Autodesk Inventor part; units mm, degrees
ref_plane "YZ Plane" through (0, 0, 0) normal (1, 0, 0) x (0, 1, 0)
ref_plane "XZ Plane" through (0, 0, 0) normal (0, 1, 0) x (-1, 0, 0)
ref_plane "XY Plane" through (0, 0, 0) normal (0, 0, 1) x (1, 0, 0)
sketch "스케치1" plane through (0, 0, 0) normal (0, 1, 0) x (-1, 0, 0)
  line L0 (-62.3615, 62.3615) -> (-22.8259, 85.1874)
  line L1 (-22.8259, 85.1874) -> (22.8259, 85.1874)
  line L2 (22.8259, 85.1874) -> (62.3615, 62.3615)
  line L3 (62.3615, 62.3615) -> (85.1874, 22.8259)
  line L4 (85.1874, 22.8259) -> (85.1874, -22.8259)
  line L5 (85.1874, -22.8259) -> (62.3615, -62.3615)
  line L6 (62.3615, -62.3615) -> (22.8259, -85.1874)
  line L7 (22.8259, -85.1874) -> (-22.8259, -85.1874)
  line L8 (-22.8259, -85.1874) -> (-62.3615, -62.3615)
  line L9 (-62.3615, -62.3615) -> (-85.1874, -22.8259)
  line L10 (-85.1874, -22.8259) -> (-85.1874, 22.8259)
  line L11 (-85.1874, 22.8259) -> (-62.3615, 62.3615)
  line L12 (88.3874, -23.6833) -> (64.7041, -64.7041)
  line L13 (64.7041, -64.7041) -> (23.6833, -88.3874)
  line L14 (23.6833, -88.3874) -> (-23.6833, -88.3874)
  line L15 (-23.6833, -88.3874) -> (-64.7041, -64.7041)
  line L16 (-64.7041, -64.7041) -> (-88.3874, -23.6833)
  line L17 (-88.3874, -23.6833) -> (-88.3874, 23.6833)
  line L18 (-88.3874, 23.6833) -> (-64.7041, 64.7041)
  line L19 (-64.7041, 64.7041) -> (-23.6833, 88.3874)
  line L20 (-23.6833, 88.3874) -> (23.6833, 88.3874)
  line L21 (23.6833, 88.3874) -> (64.7041, 64.7041)
  line L22 (64.7041, 64.7041) -> (88.3874, 23.6833)
  line L23 (88.3874, 23.6833) -> (88.3874, -23.6833)
  point P0 (0, 0)
  point P1 (0, 0)
  point P2 (0, 0)
  dimension "d0" = 176.385
  dimension "d1" = 3.2
extrude "돌출1" add sketch "스케치1" along normal blind 6.8 contours L0 L1 L2 L3 L4 L5 L6 L7 L8 L9 L10 L11 | L12 L13 L14 L15 L16 L17 L18 L19 L20 L21 L22 L23
sketch "스케치2" plane through (0, 6.8, 0) normal (0, 1, 0) x (1, 0, 0)
  line L0 (-23.2546, 86.7874) -> (23.2546, 86.7874)
  line L1 (23.2546, 86.7874) -> (63.5328, 63.5328)
  line L2 (63.5328, 63.5328) -> (86.7874, 23.2546)
  line L3 (86.7874, 23.2546) -> (86.7874, -23.2546)
  line L4 (86.7874, -23.2546) -> (63.5328, -63.5328)
  line L5 (63.5328, -63.5328) -> (23.2546, -86.7874)
  line L6 (23.2546, -86.7874) -> (-23.2546, -86.7874)
  line L7 (-23.2546, -86.7874) -> (-63.5328, -63.5328)
  line L8 (-63.5328, -63.5328) -> (-86.7874, -23.2546)
  line L9 (-86.7874, -23.2546) -> (-86.7874, 23.2546)
  line L10 (-86.7874, 23.2546) -> (-63.5328, 63.5328)
  line L11 (-63.5328, 63.5328) -> (-23.2546, 86.7874)
  line L12 (-88.3874, 23.6833) -> (-88.3874, -23.6833)
  line L13 (22.7187, -84.7874) -> (-22.7187, -84.7874)
  line L14 (-22.7187, -84.7874) -> (-62.0687, -62.0687)
  line L15 (-62.0687, -62.0687) -> (-84.7874, -22.7187)
  line L16 (-84.7874, -22.7187) -> (-84.7874, 22.7187)
  line L17 (-84.7874, 22.7187) -> (-62.0687, 62.0687)
  line L18 (-62.0687, 62.0687) -> (-22.7187, 84.7874)
  line L19 (-22.7187, 84.7874) -> (22.7187, 84.7874)
  line L20 (22.7187, 84.7874) -> (62.0687, 62.0687)
  line L21 (62.0687, 62.0687) -> (84.7874, 22.7187)
  line L22 (84.7874, 22.7187) -> (84.7874, -22.7187)
  line L23 (84.7874, -22.7187) -> (62.0687, -62.0687)
  line L24 (62.0687, -62.0687) -> (22.7187, -84.7874)
  point P0 (0, 0)
  point P1 (0, 0)
  point P2 (0, 0)
  dimension "d4" = 1.6
  dimension "d5" = 2
extrude "돌출2" cut sketch "스케치2" against normal blind 1.2
sketch "스케치5" plane through (0, 6.8, 0) normal (0, 1, 0) x (1, 0, 0)
  line L0 (-62.0687, -62.0687) -> (-22.7187, -84.7874)
  line L1 (-22.7187, -84.7874) -> (22.7187, -84.7874)
  line L2 (22.7187, -84.7874) -> (62.0687, -62.0687)
  line L3 (62.0687, -62.0687) -> (84.7874, -22.7187)
  line L4 (84.7874, -22.7187) -> (84.7874, 22.7187)
  line L5 (84.7874, 22.7187) -> (62.0687, 62.0687)
  line L6 (62.0687, 62.0687) -> (22.7187, 84.7874)
  line L7 (22.7187, 84.7874) -> (-22.7187, 84.7874)
  line L8 (-22.7187, 84.7874) -> (-62.0687, 62.0687)
  line L9 (-62.0687, 62.0687) -> (-84.7874, 22.7187)
  line L10 (-84.7874, 22.7187) -> (-84.7874, -22.7187)
  line L11 (-84.7874, -22.7187) -> (-62.0687, -62.0687)
  point P0 (0, 0)
extrude "돌출5" cut sketch "스케치5" against normal blind 0.6
fillet "모깎기1" radius 1.2 24 edges at (76.5457, 0, 44.1937) (76.5457, 6.8, 44.1937) (88.3874, 6.8, 0) (88.3874, 0, 0) (76.5457, 6.8, -44.1937) (76.5457, 0, -44.1937) (44.1937, 6.8, -76.5457) (44.1937, 0, -76.5457) (0, 0, -88.3874) (0, 6.8, -88.3874) (-44.1937, 6.8, -76.5457) (-44.1937, 0, -76.5457) (-76.5457, 0, -44.1937) (-76.5457, 6.8, -44.1937) (-88.3874, 0, 0) (-88.3874, 6.8, 0) (-76.5457, 0, 44.1937) (-76.5457, 6.8, 44.1937) (-44.1937, 0, 76.5457) (-44.1937, 6.8, 76.5457) (0, 0, 88.3874) (0, 6.8, 88.3874) (44.1937, 0, 76.5457) (44.1937, 6.8, 76.5457)
sketch "스케치7" plane through (0, 0, 0) normal (0, -1, 0) x (1, 0, 0)
  line L0 (10, -7.5) -> (-10, -7.5)
  line L1 (-10, -7.5) -> (-10, -2.5)
  line L2 (-10, -2.5) -> (10, -2.5)
  line L3 (10, -2.5) -> (10, -7.5)
  line L4 (10, -7.5) -> (-10, -2.5) construction
  line L5 (-10, -7.5) -> (10, -2.5) construction
  line L6 (0, 0) -> (-24.3026, 0)
  line L7 (10, 7.5) -> (-10, 7.5)
  line L8 (-10, 7.5) -> (-10, 2.5)
  line L9 (-10, 2.5) -> (10, 2.5)
  line L10 (10, 2.5) -> (10, 7.5)
  line L11 (10, 7.5) -> (-10, 2.5) construction
  line L12 (-10, 7.5) -> (10, 2.5) construction
  point P0 (0, -5)
  point P1 (0, 5)
  dimension "d26" = 20
  dimension "d27" = 5
  dimension "d28" = 2.5
extrude "돌출7" add sketch "스케치7" along normal blind 10
sketch "스케치8" plane through (-10, 0, 7.5) normal (0, 0, 1) x (1, 0, 0)
  circle A0 centre (15, -5) radius 1.25
  line L0 (-13.3618, 0) -> (33.3618, 0)
  line L1 (20, 0) -> (20, -10)
  line L2 (20, -10) -> (0, -10)
  line L3 (10, -10) -> (10, 0)
  circle A1 centre (5, -5) radius 1.25
  point P0 (20, -5)
  dimension "d31" = 2.5
  dimension "d32" = 5
  dimension "d33" = 5
extrude "돌출8" cut sketch "스케치8" against normal up to surface (15 mm away) contours A0 | A1
properties part number "(x2)_POSPA_Large_Bottom"
Build history of the part. All positions in model axes, mm. A direction names the side the tool comes from. Give positions to 0.01 mm unless a question says otherwise; leave off trailing zeros. Use a Markdown table: item, result.
(1) Wall check: line 1 along Y through (x, z) = (-5, 3); line 2 along Z through (x, y) = (28.5, 5.75); line 3 along Z through (x, y) = (8.5, -0.75). Give the ranges that are in metal, low to high.
Taken from the geometry:
| item | result |
|---|---|
| line 1 | -10 to -6.25, -3.75 to 6.2 |
| line 2 | -85.6 to -83.76, -81.45 to 81.45, 83.76 to 85.6 |
| line 3 | -7.5 to -2.5, 2.5 to 7.5 |
(2) Drop flat-ended pins along their axis: pin 1 Ø1.5 at (y, z) = (-3.5, 6) entering from +X; pin 2 Ø1 at (x, y) = (7.5, 6.5) entering from -Z; pin 3 Ø5 at (x, y) = (-1.5, -4) entering from +Z. Give the stop position or say it passes through.
Taken from the geometry:
| item | result |
|---|---|
| pin 1 | x = 10 |
| pin 2 | z = -88.32 |
| pin 3 | z = 7.5 |
(3) Pull direction Z, two halves, no side cores. Call faces 1 (the face through (-73.27, 5.9, 42.67)), 2 (the face through (-76.399, 0.342, 43.726)), 3 (the face through (-10, -5, 5)): +Z half, -Z half, draft (parallel to the pull), parting line (faces both ways), or undercut.
Taken from the geometry:
| item | result |
|---|---|
| face 1 | undercut |
| face 2 | +Z half |
| face 3 | draft |
(4) Which spindle directions (+Z, -Z, +X, -X, +Y, -Y) get a long thin tool onto all of the face, cutting with end or side? Do faces 4 (the face through (-43.735, 6.439, -76.415)), 5 (the face through (0, -5, 7.5)), 6 (the face through (73.27, 5.9, -42.67)). Say none if no direction does.
Taken from the geometry:
| item | result |
|---|---|
| face 4 | -Z, -X, +Y |
| face 5 | +Z, +X, -X, -Y |
| face 6 | +Y |
